Autodesk Inventor part; units mm, degrees
ref_plane "YZ Plane" through (0, 0, 0) normal (1, 0, 0) x (0, 1, 0)
ref_plane "XZ Plane" through (0, 0, 0) normal (0, 1, 0) x (-1, 0, 0)
ref_plane "XY Plane" through (0, 0, 0) normal (0, 0, 1) x (1, 0, 0)
sketch "Boceto1" plane through (0, 0, 0) normal (0, 0, 1) x (1, 0, 0)
  circle A0 centre (0, 0) radius 17.5
  circle A1 centre (0, 0) radius 15.5
  dimension "d0" = 35
  dimension "d1" = 31
extrude "Extrusión1" add sketch "Boceto1" along normal blind 2
sketch "Boceto2" plane through (0, 0, 2) normal (0, 0, 1) x (1, 0, 0)
  circle A0 centre (0, 0) radius 17.5
extrude "Extrusión2" add sketch "Boceto2" along normal blind 2
sketch "Boceto3" plane through (0, 0, 2) normal (0, 0, -1) x (-1, 0, 0)
  circle A0 centre (0, 0) radius 15.5
  circle A1 centre (0, 0) radius 15.5
  circle A2 centre (0, 0) radius 14
  circle A3 centre (0, 0) radius 12.5
  circle A4 centre (0, 0) radius 11
  circle A5 centre (0, 0) radius 9.5
  circle A6 centre (0, 0) radius 8
  circle A7 centre (0, 0) radius 6.5
  circle A8 centre (0, 0) radius 5
  circle A9 centre (0, 0) radius 3.5
  circle A10 centre (0, 0) radius 2
  line L0 (-0.5014, 1.9361) -> (-0.5014, 2)
  line L1 (-0.5014, 1.9361) -> (-0.5014, 15.5)
  line L2 (-0.5014, 1.9361) -> (13.0625, 1.9361) construction
  line L3 (0.5019, 1.9361) -> (0.5019, 15.5)
  line L4 (0.5019, 1.9361) -> (0.5019, -15.5)
  line L5 (-0.5014, 1.9361) -> (-0.5014, -15.5)
  line L6 (1.9361, 0.5016) -> (15.5, 0.5016)
  line L7 (1.9361, -0.5011) -> (15.5, -0.5011)
  line L8 (1.9361, -0.5011) -> (-15.5, -0.5011)
  line L9 (1.9361, 0.5016) -> (-15.5, 0.5016)
  dimension "d7" = 28
  dimension "d8" = 25
  dimension "d9" = 22
  dimension "d10" = 19
  dimension "d11" = 16
  dimension "d12" = 13
  dimension "d13" = 10
  dimension "d14" = 7
  dimension "d15" = 4
  dimension "d16" = 90
extrude "Extrusión3" cut sketch "Boceto3" against normal blind 2 contours A0 L7 A2 L6 | L6 A2 L3 A0 | A0 L4 A2 L7 | L3 A2 L1 A0 | A0 L5 A2 L4 | L1 A2 L9 A0 | L6 A4 L3 A3 | A3 L7 A4 L6 | A0 L8 A2 L5 | A3 L4 A4 L7 | L9 A2 L8 A0 | L3 A4 L1 A3 | A3 L5 A4 L4 | L1 A4 L9 A3 | L6 A6 L3 A5 | A5 L7 A6 L6 | A3 L8 A4 L5 | A5 L4 A6 L7 | L9 A4 L8 A3 | L3 A6 L1 A5 | A5 L5 A6 L4 | L1 A6 L9 A5 | L6 A8 L3 A7 | A7 L7 A8 L6 | A5 L8 A6 L5 | A7 L4 A8 L7 | L9 A6 L8 A5 | L3 A8 L1 A7 | A7 L5 A8 L4 | L1 A8 L9 A7 | L6 A10 L3 A9 | A9 L7 A10 L6 | A7 L8 A8 L5 | A9 L4 A10 L7 | L9 A8 L8 A7 | L3 A10 L0 L1 A9 | A9 L5 A10 L4 | L1 L0 A10 L9 A9 | A9 L8 A10 L5 | L9 A10 L8 A9
sketch "Boceto4" plane through (0, 0, 4) normal (0, 0, 1) x (1, 0, 0)
  line L0 (-16.1458, 0.5) -> (16.1458, 0.5)
  line L1 (16.1458, 0.5) -> (16.1458, -0.5)
  line L2 (16.1458, -0.5) -> (-16.1458, -0.5)
  line L3 (-16.1458, -0.5) -> (-16.1458, 0.5)
  line L4 (-16.1458, 0.5) -> (16.1458, -0.5) construction
  line L5 (16.1458, 0.5) -> (-16.1458, -0.5) construction
  line L6 (-0.5, -16.1458) -> (0.5, -16.1458)
  line L7 (0.5, -16.1458) -> (0.5, 16.1458)
  line L8 (0.5, 16.1458) -> (-0.5, 16.1458)
  line L9 (-0.5, 16.1458) -> (-0.5, -16.1458)
  line L10 (-0.5, -16.1458) -> (0.5, 16.1458) construction
  line L11 (0.5, -16.1458) -> (-0.5, 16.1458) construction
  point P0 (0, 0)
  point P1 (0, 0)
  dimension "d19" = 1
  dimension "d20" = 1
extrude "Extrusión4" add sketch "Boceto4" against normal blind 2
equation "\"Radio_pliegue\" = Grosor"
equation "\"Anchura_desahogo_plegado\" = Grosor"
equation "\"Profundidad_desahogo_plegado\" = 0.5 * Grosor"
equation "\"Tamaño_destalonado\" = 4 * Grosor"
equation "\"Remanente_mínimo\" = 2 * Grosor"
equation "\"Radiodetransición\" = Radio_pliegue"
equation "\"Tamaño_de_radio_de_Jacobi\" = Radio_pliegue"
equation "\"TamañoSeparación\" = Grosor"
properties part number "Lattice 2"
Read the model definition and answer for the solid it produces. Units are mm, in the model's axes. Give positions to 0.01 mm unless a question says otherwise; leave off trailing zeros. Write each loop counter-clockwise with the first axis right and the second up, starting at its lowest first coordinate (ties: lowest second). Pieces come first, ordered by that corner, then holes. Notation, with made-up numbers: (20, 21.25) - (65, 21.25) arc R21 ccw to (65, 36.25) - close; hole circle Ø10 at (21.5, 88). An arc over 180 degrees is marked (long way). Write item = value, one per line. Start each with the question number.
Item 1: Find the intervals of material crossed by probe 1 along Y at (x, z) = (10, 3.15); probe 2 along Y at (x, z) = (0, 1.25); probe 3 along Y at (x, z) = (11.5, 2.65), in increasing order. Write a range as [from, to].
Item 2: Find section D-D (z = 0.75). Give the vertices of the cut face in (x, y).
Item 3: Each of these flat-tipped pins is pushed along its axis until it touches: P1, Ø0.8, axis at y = -8.5, z = 3, coming from the -X side; P2, Ø0.5, axis at y = 3, z = 3.5, coming from the +X side; P3, Ø1, axis at x = 8.5, z = 3, coming from the +Y side. Where does it stop, or does it pass through?
Item 4: Find section A-A (x = -9). Give the vertices of the cut face in (y, z).
Item 5: The mould has two halves that part along X. Classify faces 1 (the cylindrical face through (-7.697, -7.858, 2.986)), 2 (the flat face through (3, 0.5, 3)), 3 (the flat face through (-7, -14, 0)): +X half, -X half, draft (parallel to the pull), parting line (faces both ways), or undercut.
Item 6: Find section B-B (y = 0). Give the vertices of the cut face in (x, z), then the cut area to 3 significant figures.
Response:
q1.probe_1 = [-14.36, -11.84], [-9.8, -7.5], [-4.58, 4.58], [7.5, 9.8], [11.84, 14.36]
q1.probe_2 = [-17.5, -15.5], [15.5, 17.5]
q1.probe_3 = [-13.19, -10.39], [-7.98, -4.9], [-0.5, 0.5], [4.9, 7.98], [10.39, 13.19]
q2.outline = circle Ø35 at (0, 0); hole circle Ø31 at (0, 0)
q3.P1 = -15.51
q3.P2 = 17.28
q3.P3 = 15.56
q4.outline = (-15.01, 0) - (-12.62, 0) - (-12.62, 4) - (-15.01, 4) - close; (-10.72, 2) - (-8.67, 2) - (-8.67, 4) - (-10.72, 4) - close; (-6.32, 2) - (-3.04, 2) - (-3.04, 4) - (-6.32, 4) - close; (-0.5, 2) - (0.5, 2) - (0.5, 4) - (-0.5, 4) - close; (3.04, 2) - (6.32, 2) - (6.32, 4) - (3.04, 4) - close; (8.67, 2) - (10.72, 2) - (10.72, 4) - (8.67, 4) - close; (12.62, 0) - (15.01, 0) - (15.01, 4) - (12.62, 4) - close
q5.face_1 = undercut
q5.face_2 = undercut
q5.face_3 = draft
q6.outline = (-17.5, 0) - (-15.5, 0) - (-15.5, 2) - (15.5, 2) - (15.5, 0) - (17.5, 0) - (17.5, 4) - (-17.5, 4) - close
q6.area = 78.0 mm²
